Check sheet for the modelled part. Datum: model origin and axes. Units: mm. A direction names the side the tool comes from. Give positions to 0.01 mm unless a question says otherwise; leave off trailing zeros. Order: outer loops, then holes, each group sorted by start corner. A loop starts at its lowest first (then second) coordinate and runs counter-clockwise, first axis right, second up.
Autodesk Inventor part; units mm, degrees
ref_plane "YZ Plane" through (0, 0, 0) normal (1, 0, 0) x (0, 1, 0)
ref_plane "XZ Plane" through (0, 0, 0) normal (0, 1, 0) x (-1, 0, 0)
ref_plane "XY Plane" through (0, 0, 0) normal (0, 0, 1) x (1, 0, 0)
sketch "Sketch1" plane through (0, 0, 0) normal (0, 1, 0) x (-1, 0, 0)
  point P0 (0, 0)
sketch "Sketch2" plane through (0, 0, 0) normal (0, 1, 0) x (-1, 0, 0)
  line L0 (5.25, 12.5) -> (-5.25, 12.5)
  line L1 (-5.25, 12.5) -> (-5.25, -12.5)
  line L2 (-5.25, -12.5) -> (5.25, -12.5)
  line L3 (5.25, -12.5) -> (5.25, 12.5)
  point P0 (0, 0)
  dimension "d0" = 10.5
  dimension "d1" = 25
  dimension "d2" = 12.5
  dimension "d3" = 5.25
extrude "Extrusion1" add sketch "Sketch2" along normal blind 12.5
sketch "Sketch3" plane through (0, 12.5, 0) normal (0, 1, 0) x (1, 0, 0)
  line L0 (-2.25, -4.75) -> (2.25, -4.75)
  line L1 (2.25, -4.75) -> (2.25, 4.75)
  line L2 (2.25, 4.75) -> (-2.25, 4.75)
  line L3 (-2.25, 4.75) -> (-2.25, -4.75)
  line L4 (-2.25, -4.75) -> (-3.75, -4.75)
  line L5 (-3.75, -4.75) -> (-3.75, 4.75)
  line L6 (-3.75, 4.75) -> (-2.25, 4.75)
  line L7 (-2.25, 4.75) -> (-2.25, -4.75)
  line L8 (2.25, 4.75) -> (3.75, 4.75)
  line L9 (3.75, 4.75) -> (3.75, -4.75)
  line L10 (3.75, -4.75) -> (2.25, -4.75)
  line L11 (2.25, -4.75) -> (2.25, 4.75)
  circle A0 centre (0, -10) radius 0.75
  circle A1 centre (0, 10) radius 0.75
  line L12 (-5.25, -12.5) -> (5.25, -12.5)
  line L13 (5.25, 12.5) -> (-5.25, 12.5)
  line L14 (-2, -11.5) -> (2, -11.5)
  line L15 (2, -11.5) -> (2, -8.5)
  line L16 (2, -8.5) -> (-2, -8.5)
  line L17 (-2, -8.5) -> (-2, -11.5)
  line L18 (-2, 8.5) -> (2, 8.5)
  line L19 (2, 8.5) -> (2, 11.5)
  line L20 (2, 11.5) -> (-2, 11.5)
  line L21 (-2, 11.5) -> (-2, 8.5)
  line L22 (-2, -11.5) -> (-3.75, -4.75)
  line L23 (-3.75, 4.75) -> (-2, 11.5)
  line L24 (2, 11.5) -> (3.75, 4.75)
  line L25 (3.75, -4.75) -> (2, -11.5)
  point P0 (0, 0)
  dimension "d6" = 4.5
  dimension "d7" = 9.5
  dimension "d8" = 4.75
  dimension "d9" = 2.25
  dimension "d10" = 1.5
  dimension "d11" = 1.5
  dimension "d12" = 1.5
  dimension "d13" = 1.5
  dimension "d14" = 2.5
  dimension "d15" = 2.5
  dimension "d16" = 4
  dimension "d17" = 3
  dimension "d18" = 4
  dimension "d19" = 3
  dimension "d20" = 1.5
  dimension "d21" = 2
  dimension "d22" = 2
  dimension "d23" = 1.5
extrude "Extrusion2" add sketch "Sketch3" along normal blind 1 contours L4 L5 L6 L3 | L0 L10 L25 L15 L16 L17 L22 L4 | L1 L8 L9 L10 | L6 L23 L21 L18 L19 L24 L8 L2 | L17 L16 L15 L14 | L20 L19 L18 L21
sketch "Sketch4" plane through (0, 12.5, 0) normal (0, 1, 0) x (1, 0, 0)
  line L0 (-1.95, -4.45) -> (1.95, -4.45)
  line L1 (1.95, -4.45) -> (1.95, 0.05)
  line L2 (1.95, 0.05) -> (-1.95, 0.05)
  line L3 (-1.95, 0.05) -> (-1.95, -4.45)
  line L4 (2.25, -4.75) -> (-2.25, -4.75)
  line L5 (-2.25, -4.75) -> (-2.25, 4.75)
  line L6 (2.25, 4.75) -> (2.25, -4.75)
  point P0 (0, 0)
  dimension "d26" = 0.3
  dimension "d27" = 0.3
  dimension "d28" = 0.3
  dimension "d29" = 4.5
extrude "Extrusion3" add sketch "Sketch4" along normal blind 4
sketch "Sketch5" plane through (0, 0, 0) normal (0, -1, 0) x (1, 0, 0)
  line L0 (4.5, 8.5) -> (-4.5, 8.5)
  line L1 (-4.5, 8.5) -> (-4.5, -8.5)
  line L2 (-4.5, -8.5) -> (4.5, -8.5)
  line L3 (4.5, -8.5) -> (4.5, 8.5)
  point P0 (0, 0)
  dimension "d32" = 9
  dimension "d33" = 17
  dimension "d34" = 8.5
  dimension "d35" = 4.5
extrude "Extrusion4" add sketch "Sketch5" along normal blind 2
chamfer "Chamfer1" distance 1 angle 45 4 edges at (0, -2, 8.5) (4.5, -2, 0) (0, -2, -8.5) (-4.5, -2, 0)
fillet "Fillet1" radius 0.5 8 edges at (0, 13.5, 11.5) (-2.875, 13.5, 8.125) (2.875, 13.5, 8.125) (-3.75, 13.5, 0) (-2.875, 13.5, -8.125) (0, 13.5, -11.5) (2.875, 13.5, -8.125) (3.75, 13.5, 0)
fillet "Fillet2" radius 0.25 4 edges at (-5.25, 12.5, 0) (0, 12.5, 12.5) (5.25, 12.5, 0) (0, 12.5, -12.5)
equation "\"d20\" = 0.5 * d17"
equation "\"d21\" = 0.5 * d16"
equation "\"d22\" = 0.5 * d18"
equation "\"d23\" = 0.5 * d19"
properties part number "switch"
1) Draft check along X on faces 4 (the face through (4, 12.5, -1)), 5 (the face through (2.25, 13, 0)), 6 (the face through (-4, -1.5, -0.1)). Enter one of: +X half, -X half, draft (parallel to the pull), parting line (faces both ways), or undercut.
Recorded:
face 4: draft
face 5: undercut
face 6: -X half
2) Depth check by flat-ended pin: pin 1 Ø0.5 at (x, y) = (-2, -0.5) entering from -Z; pin 2 Ø0.8 at (y, z) = (-0.5, 4) entering from +X; pin 3 Ø4 at (x, z) = (-3, 5.5) entering from +Y; pin 4 Ø0.5 at (x, y) = (-0.5, -0.5) entering from +Z. Enter the tip coordinate at first touch or a pass-through.
Recorded:
pin 1: stops at z = -8.5
pin 2: stops at x = 4.5
pin 3: stops at y = 16.5
pin 4: stops at z = 8.5
3) Section check B-B, the plane z = -1.25. Record the cut outline in (x, y), then the cut area to 3 significant figures.
Recorded:
outline: (-5.25, 0) - (-4.5, 0) - (-4.5, -1) - (-3.5, -2) - (3.5, -2) - (4.5, -1) - (4.5, 0) - (5.25, 0) - (5.25, 12.25) arc R0.25 ccw to (5, 12.5) - (3.75, 12.5) - (3.75, 13) arc R0.5 ccw to (3.25, 13.5) - (2.25, 13.5) - (2.25, 12.5) - (-2.25, 12.5) - (-2.25, 13.5) - (-3.25, 13.5) arc R0.5 ccw to (-3.75, 13) - (-3.75, 12.5) - (-5, 12.5) arc R0.25 ccw to (-5.25, 12.25) - close
area: 151 mm2
4) Set-up check for faces 1 (the face through (0, 13, 4.75)), 2 (the face through (2.887, 12.746, 8.078)), 3 (the face through (2.863, 12.746, -8.172)): record each of +Z, -Z, +X, -X, +Y, -Y from which the full face is reachable in a straight line by a thin tool's end or side.
Recorded:
face 1: +Y
face 2: +Z, +X, +Y
face 3: -Z, +X, +Y
5) Material ranges on L1, parallel to Z at x = 0, y = 12.95; L2, parallel to X at y = 15, z = 1.75; L3, parallel to Y at x = 1, z = 11.75, recorded low to high.
Recorded:
L1: z = -11.5 to -10.75, -9.25 to -4.75, -0.05 to 4.45, 4.75 to 9.25, 10.75 to 11.5
L2: x = -1.95 to 1.95
L3: y = 0 to 12.5
